The drawing under review shows one solid part. Ordinate dimensions are in mm from its lowest x, y, z. A direction names the side the tool comes from. Give positions to 0.01 mm unless a question says otherwise; leave off trailing zeros. Write each loop counter-clockwise with the first axis right and the second up, starting at its lowest first coordinate (ties: lowest second). Pieces come first, ordered by that corner, then holes. Notation, with made-up numbers: M 8.25,73.25 L 66.25,73.25 A32 ccw 66.25,106.25 Z; hole C 19,73.5 d7. An arc over 180 degrees is marked long. Answer as a JSON object with one key per item and string values. Group by question number.
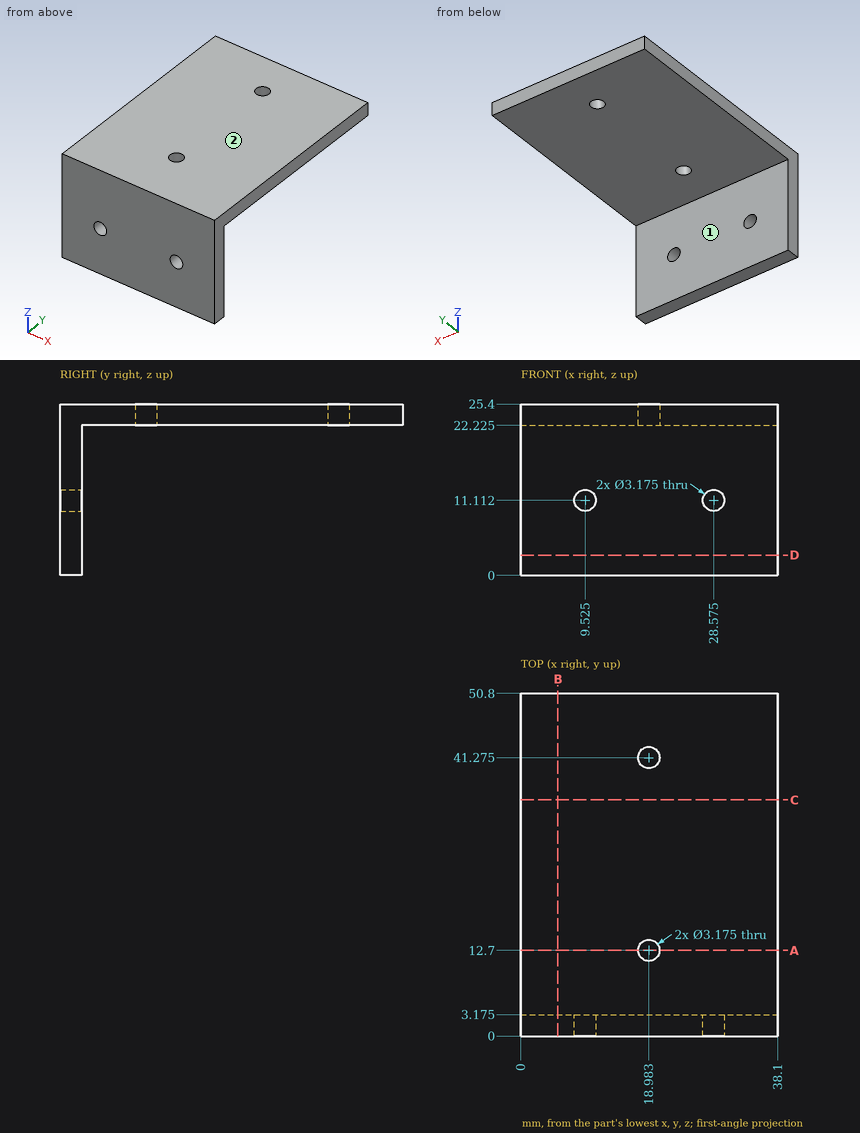
Item 1: Machinability: for the marked faces 1 and 2, which of the approach directions +Z, -Z, +X, -X, +Y, -Y give a long, thin tool a straight path to every point of the face, cutting with its end or side? Answer none if there is none.
Item 2: Consider section D-D (z = 3). Give the boundary of the cut face in (x, y) (1 decimal), plus the area to 3 significant figures.
Item 3: Consider section B-B (x = 5.5). Give the boundary of the cut face in (y, z) (1 decimal), plus the area to 3 significant figures.
Item 4: Consider section A-A (y = 12.7). Give the boundary of the cut face in (x, z) (1 decimal), plus the area to 3 significant figures.
Item 5: To check wall thickness, follow probe 1 along Z at (x, y) = (32, 46) (1 decimal); probe 2 along Y at (x, z) = (17, 11.5) (1 decimal). State the ranges of each line that lie inside material, in increasing order.
Item 6: Insertion check: P1, Ø10, axis at x = 20, z = 13.5, coming from the +Y side (1 decimal); P2, Ø1.5, axis at x = 19.5, y = 19, coming from the -Z side (1 decimal). Each pin has a flat end and moves straight along its axis. Give the tip position at first contact, or say it passes through.
Item 7: Consider section C-C (y = 35). Give the boundary of the cut face in (x, z) (1 decimal), plus the area to 3 significant figures.
Result set:
{
 "1": {"face 1": "-Z, +X, -X, +Y", "face 2": "+Z, +X, -X, +Y, -Y"},
 "2": {"outline": "M 0,0 L 38.1,0 L 38.1,3.2 L 0,3.2 Z", "area": "121 mm^2"},
 "3": {"outline": "M 0,0 L 3.2,0 L 3.2,22.2 L 50.8,22.2 L 50.8,25.4 L 0,25.4 Z", "area": "232 mm^2"},
 "4": {"outline": "M 0,22.2 L 17.4,22.2 L 17.4,25.4 L 0,25.4 Z; M 20.6,22.2 L 38.1,22.2 L 38.1,25.4 L 20.6,25.4 Z", "area": "111 mm^2"},
 "5": {"probe 1": "z = 22.2 to 25.4", "probe 2": "y = 0 to 3.2"},
 "6": {"P1": "stops at y = 3.2", "P2": "stops at z = 22.2"},
 "7": {"outline": "M 0,22.2 L 38.1,22.2 L 38.1,25.4 L 0,25.4 Z", "area": "121 mm^2"}
}
